Geometry: final body of the model. Coordinates: model frame, mm. A direction names the side the tool comes from. Give positions to 0.01 mm unless a question says otherwise; leave off trailing zeros. Write each loop counter-clockwise with the first axis right and the second up, starting at its lowest first coordinate (ties: lowest second). Pieces come first, ordered by that corner, then holes. Notation, with made-up numbers: (-9.5, 77) -> (-4.5, 77) arc R23 ccw to (-4.5, 95) -> close; hole circle Ø11 at (66, 48). An arc over 180 degrees is marked (long way). Use CSV: the item, a comma, the result in double quotes. Start each with the question number.
1) Draft query along Z for faces 3 (the face through (8.1, 6.5, -9.8)), 4 (the face through (4.23, 1.47, 7.66)), 5 (the face through (8, 6.662, -7)). Return one class per face: pulls with the +Z half, pulls with the -Z half, needs draft (parallel to the pull), parting line crosses it, or undercut.
2) Material intervals for line 1 (X direction, y = -0.25, z = 7.25); line 2 (X direction, y = -0.5, z = 7.75); line 3 (Z direction, x = 10.5, y = 4.75), sorted ascending. Write a range as [from, to].
3) Set-up query: faces 1 (the face through (0.57, 0.9, -0.63)), 2 (the face through (8.11, 1.31, 14.71)). Return all of +Z, -Z, +X, -X, +Y, -Y with unobstructed straight access to the full face (end or side cutting, diameter ignored); none if empty.
4) Contact query for flat-ended pins moving along their axis: P1, Ø1, axis at x = 11, z = 10.5, coming from the +Y side; P2, Ø6, axis at x = 5, z = -1, coming from the +Y side; P3, Ø1.5, axis at y = 0.5, z = 3.5, coming from the -X side. Output: stop coordinate, or through.
5) Section A-A (x = 6.5). Output: boundary loops of the cut face in (y, z).
6) Section B-B (x = 12.75). Output: boundary loops of the cut face in (y, z).
7) Section D-D (z = 3.5). Output: boundary loops of the cut face in (x, y).
8) Section C-C (y = 2.75). Count the separate pieces of the cut face and the enclosed holes in it, plus the area to 3 significant figures.
```python
from build123d import *

# Parameters (mm, degrees)
F1_DEPTH = 16
F2_R     = 1.05
F3_DEPTH = 7.7105812745
F4_R     = 2


with BuildPart() as f1:
    # F0 (on Right) → F1 (new body)
    with BuildSketch(Plane.YZ):
        Polygon((-1.5, -15), (1.5, -15), (1.5, -7), (1.5, -3), (1.5, 5.2020410289), (1.5, 15), (-1.5, 15), align=None)
        Polygon((6.5, 5.2020410289), (1.5, 15), (1.5, 5.2020410289), align=None)
        Polygon((1.5, -7), (1.5, -15), (6.6618086312, -9.8381913688), (6.6618086312, -4.7058628306), (5.187990124, -5.3608932782), align=None)
    extrude(amount=F1_DEPTH)

    # F2 (on face) → F3 (cut, up to face)
    with BuildSketch(Plane(origin=(0, 7.2631977094, 3.7064850602), x_dir=(-1, 0, 0), z_dir=(0, 0.8907235428, 0.4545454545))):
        with Locations((-12, 7.1790349606)):
            Circle(F2_R)
        with Locations((-4, 7.1790349606)):
            Circle(F2_R)
    extrude(amount=-F3_DEPTH, mode=Mode.SUBTRACT)

    # F4
    f4_edges = [f1.edges().sort_by_distance(p)[0] for p in [
        (16, 1.5, -0.898979),
        (0, 1.5, -0.898979),
        (16, 4, 10.101021),
        (0, 4, 10.101021),
        (8, 6.5, 5.202041),
        (8, 6.661809, -9.838191),
        (16, 4.080904, -12.419096),
        (0, 4.080904, -12.419096),
        (16, 4.080904, -5.852931),
        (0, 4.080904, -5.852931),
        (8, 1.5, 15),
        (8, 1.5, -15),
    ]]
    fillet(f4_edges, radius=F4_R)


solid = f1.part
```
Answers follow:
1,face 3,"pulls with the -Z half"
1,face 4,"undercut"
1,face 5,"needs draft"
2,line 1,"x = [0, 3.14], [4.86, 11.14], [12.86, 16]"
2,line 2,"x = [0, 2.95], [5.05, 10.95], [13.05, 16]"
2,line 3,"z = [-11.75, -5.56], [5.9, 8.63]"
3,face 1,"-X"
3,face 2,"+Z, +X, -X, +Y"
4,P1,"stops at y = 4.05"
4,P2,"stops at y = 1.5"
4,P3,"stops at x = 0.02"
5,outline,"(-1.5, -15) -> (0.67, -15) arc R2 ccw to (2.09, -14.41) -> (6.08, -10.42) arc R2 ccw to (6.66, -9.01) -> (6.66, -4.71) -> (1.5, -7) -> (1.5, 5.2) -> (3.23, 5.2) arc R2 ccw to (5.02, 8.11) -> (2.06, 13.91) arc R2 ccw to (0.28, 15) -> (-1.5, 15) -> close"
6,outline,"(-1.5, -15) -> (0.67, -15) arc R2 ccw to (2.09, -14.41) -> (6.08, -10.42) arc R2 ccw to (6.66, -9.01) -> (6.66, -4.71) -> (1.5, -7) -> (1.5, 5.2) -> (3.23, 5.2) arc R2 ccw to (5.02, 8.11) -> (4.33, 9.45) -> (-1.5, 6.47) -> close; (-1.5, 8.12) -> (3.67, 10.76) -> (2.06, 13.91) arc R2 ccw to (0.28, 15) -> (-1.5, 15) -> close"
7,outline,"(0, -1.5) -> (16, -1.5) -> (16, -0.5) arc R2 ccw to (14, 1.5) -> (2, 1.5) arc R2 ccw to (0, -0.5) -> close"
8,separate pieces,"2"
8,enclosed holes,"2"
8,area,"219 mm^2"
